Autodesk Inventor part; units mm, degrees
ref_plane "Work Plane1" through (30.1625, 0, 0) normal (0, 0, -1) x (1, 0, 0)
ref_plane "YZ Plane" through (0, 0, 0) normal (1, 0, 0) x (0, 1, 0)
ref_plane "XZ Plane" through (0, 0, 0) normal (0, 1, 0) x (-1, 0, 0)
sketch "Эскиз1" plane through (0, 0, 0) normal (0, 0, 1) x (1, 0, 0)
  line L0 (-1.3, 0) -> (5, 0)
  line L1 (5, 0) -> (5, 1)
  line L2 (5, 1) -> (0.4, 1)
  line L3 (0.4, 1) -> (0.1546, 1)
  line L4 (0.1546, 1) -> (0, 1)
  line L5 (0, 1) -> (0, 1.9)
  line L6 (-2.56, 0) -> (6.26, 0)
  line L7 (0, -0.38) -> (0, 2.28)
  line L8 (-1.3, 0) -> (-1.3, 1.9)
  line L9 (0, 1.9) -> (-1.3, 1.9)
  dimension "d0" = 5
  dimension "d1" = 4.6
  dimension "d2" = 0.2454
  dimension "d3" = 1.3
  dimension "d4" = 2
  dimension "d5" = 2
  dimension "d9" = 3.8
  dimension "d10" = 0
revolve "Базовый элемент" add sketch "Эскиз1" angle 360 about axis through (-1.3, 0, 0) along (1, 0, 0)
sketch "Эскиз2" plane through (-1.3, 0, 0) normal (-1, 0, 0) x (0, 0, 1)
  circle A0 centre (0, 0) radius 1.9
  line L0 (0, 0) -> (0, 1.9)
  line L1 (-1.9, 0.2275) -> (1.9, 0.2275)
  line L2 (1.9, 0.2275) -> (1.9, -0.2275)
  line L3 (1.9, -0.2275) -> (-1.9, -0.2275)
  line L4 (-1.9, -0.2275) -> (-1.9, 0.2275)
  line L5 (-1.9, 0) -> (1.9, 0) construction
  line L6 (0, 0.2275) -> (0, -0.2275) construction
  dimension "d11" = 0.455
  dimension "d12" = 3.8
fillet "Сопряжение1" radius 0.01 1 edges at (-1.3, -1.9, 0)
extrude "Паз" cut sketch "Эскиз2" against normal blind 0.91 contours A0 L3 L1 | L2 L3 A0 | A0 L1 L2 | L3 L4 A0 | A0 L4 L1
thread "Резьба"
chamfer "Chamfer4" distance 0.2 angle 45 1 edges at (5, -1, 0)
ref_plane "Work Plane1" through (30.1625, 0, 0) normal (0, 0, -1) x (1, 0, 0)
equation "\"d11\" = SBR"
equation "\"d12\" = KOD"
equation "\"d13\" = RR"
equation "\"d16\" = STI"
equation "\"d14\" = GEL"
equation "\"d40\" = 0.1 * GD"
equation "\"d0\" = NLG"
equation "\"d1\" = GEL"
equation "\"d2\" = GAL"
equation "\"d3\" = KOH"
equation "\"d4\" = GD"
equation "\"d5\" = BDM"
equation "\"d9\" = KOD"
equation "\"GD\" = NND"
equation "\"NLG\" = 5"
equation "\"GEL\" = 4.6"
equation "\"KOD\" = 3.8"
equation "\"KOH\" = 1.3"
equation "\"GAL\" = 0.61345 * PTC"
equation "\"BDM\" = NND"
equation "\"RR\" = 0.01"
equation "\"SBR\" = 0.455"
equation "\"STI\" = 0.91"
equation "\"KEWI\" = 0"
equation "\"GUL\" = 0.61345 * PTC"
equation "\"SPD\" = NND - 1.2269 * PTC"
equation "\"PTC\" = 0.4"
equation "\"THREADDIA\" = 2"
equation "\"TOA\" = 30deg"
equation "\"FAWI\" = 45deg"
equation "\"NND\" = 2"
equation "\"GD1\" = THREADDIA - 1.2269 * PTC"
properties part number "Винт M2-6gx5 ГОСТ 1491-80" material "Сталь, мягкая"
The listing builds one solid part. Answer for the finished solid, in the listing's coordinates (mm). A direction names the side the tool comes from. Round coordinates to 2 decimals unless told otherwise and drop trailing zeros. Loops run counter-clockwise (first coordinate to the right, second up) from the corner with the lowest first, then second, coordinate; pieces in that order, holes last. Notation, with made-up numbers: (16, -26.5) - (30, -26.5) arc R5 cw to (30, -21.5) - close; hole circle Ø5 at (25, -2). An arc over 180 degrees is marked (long way). Return JSON: item names as keys, results as strings. Group by question number.
1. Consider probe 1 along X at (y, z) = (0.5, 1.4); probe 2 along X at (y, z) = (0.15, -0.6); probe 3 along Z at (x, y) = (3, 0). Determine where each line is inside the solid, lowest interval first.
2. The part is cut by section C-C on x = 1.25. Determine the outline of the cut face in (y, z).
3. Which of the six approach directions +Z, -Z, +X, -X, +Y, -Y give full straight-line access (tool end or side, diameter ignored) to faces 1 (the flat face through (-1, 0.228, 0)), 2 (the cylindrical face through (2, 0, 1)), 3 (the flat face through (-1.3, -1, 0))?
4. The part is cut by section A-A on y = 0. Determine the outline of the cut face in (x, z), then the cut area to 3 significant figures.
5. Each of these flat-tipped pins is pushed along its axis until it touches: P1, Ø2, axis at x = -0.5, z = -1.5, coming from the +Y side; P2, Ø0.7, axis at x = -0.5, z = 0.5, coming from the +Y side; P3, Ø0.7, axis at x = -1, z = 0.5, coming from the -Y side. Where does it stop, or does it pass through?
6. The mould has two halves that part along Y. Classify faces 4 (the cylindrical face through (-0.65, -1.9, -0.08)), 5 (the flat face through (5, 0, 0)), 6 (the flat face through (-1, -0.228, 0)): pulls with the +Y half, pulls with the -Y half, needs draft (parallel to the pull), parting line crosses it, or undercut.
Resolved:
{
 "1": {"probe 1": "x = -1.3 to 0", "probe 2": "x = -0.39 to 5", "probe 3": "z = -1 to 1"},
 "2": {"outline": "circle Ø2 at (0, 0)"},
 "3": {"face 1": "+Z, -Z, -X", "face 2": "+X", "face 3": "+Z, -Z, -X, +Y, -Y"},
 "4": {"outline": "(-0.39, -1.9) - (0, -1.9) - (0, -1) - (4.8, -1) - (5, -0.8) - (5, 0.8) - (4.8, 1) - (0, 1) - (0, 1.9) - (-0.39, 1.9) - close", "area": "11.4 mm²"},
 "5": {"P1": "stops at y = 1.83", "P2": "stops at y = 1.89", "P3": "stops at y = -1.89"},
 "6": {"face 4": "parting line crosses it", "face 5": "needs draft", "face 6": "undercut"}
}
